```python
from build123d import *

# Parameters (mm, degrees)
BOSS_EXTRUDE1_DEPTH = 38.1
SKETCH2_W           = 19
SKETCH2_H           = 50
CUT_EXTRUDE1_DEPTH  = 2
CUT_EXTRUDE2_DEPTH  = 20


with BuildPart() as part:
    # Sketch1 → Boss-Extrude1 (new body)
    with BuildSketch(Plane(origin=(0, 0, 0), x_dir=(1, 0, 0), z_dir=(0, 1, 0))):
        Polygon((-138.61, 294.305), (350, -194.305), (350, -294.305), (-350, -294.305), (-350, 294.305), align=None)
    extrude(amount=BOSS_EXTRUDE1_DEPTH)

    # Sketch2 → Cut-Extrude1 (cut)
    with BuildSketch(Plane.XZ):
        with Locations((-340.5, -129.305)):
            Rectangle(SKETCH2_W, SKETCH2_H)
        with Locations((-340.5, 129.305)):
            Rectangle(SKETCH2_W, SKETCH2_H)
    extrude(amount=-CUT_EXTRUDE1_DEPTH, mode=Mode.SUBTRACT)

    # Sketch3 → Cut-Extrude2 (cut)
    with BuildSketch(Plane(origin=(0, 0, 0), x_dir=(1, 0, 0), z_dir=(0, 1, 0))):
        Polygon((-138.61, 294.305), (-181.946540118, 250.968459882), (-146.706941406, 216.891522613), (-104.668874503, 260.363874503), align=None)
    extrude(amount=CUT_EXTRUDE2_DEPTH, mode=Mode.SUBTRACT)


solid = part.part
```
CAD build for the part. Positions are in the model's coordinates, mm. A direction names the side the tool comes from. Round coordinates to 2 decimals unless told otherwise and drop trailing zeros. Write each loop counter-clockwise with the first axis right and the second up, starting at its lowest first coordinate (ties: lowest second). Pieces come first, ordered by that corner, then holes. Notation, with made-up numbers: (22.5, -18.5) -> (77.5, -18.5) arc R12 cw to (77.5, 2.5) -> close; hole circle Ø6 at (85, 81). An arc over 180 degrees is marked (long way). Answer in a Markdown table with one row per item. Add a question column.
Item 1: Drop flat-ended pins along their axis: pin 1 Ø10 at (y, z) = (19, -12.5) entering from +X (3 decimals); pin 2 Ø12 at (y, z) = (19, -177) entering from +X (3 decimals); pin 3 Ø1.6 at (y, z) = (1, 136.5) entering from -X. Give the stop position or say it passes through.
Item 2: Which spindle directions (+Z, -Z, +X, -X, +Y, -Y) get a long thin tool onto all of the face, cutting with end or side? Do faces 5 (the face through (-159.975, 9.86, -272.94)), 6 (the face through (-73, 0, 61)), 7 (the face through (-341, 2, 130)). Say none if no direction does.
Item 3: Mould opens along X. For faces 1 (the face through (102.275, 18.783, -53.42)), 2 (the face through (-164.573, 9.86, -234.169)), 3 (the face through (-350, 19, 4)), 4 (the face through (-246, 19, -294.305)) say: pulls with the +X half, pulls with the -X half, needs draft (parallel to the pull), parting line crosses it, or undercut.
Item 4: Saw through at D-D, the plane z = 0.5. Write the cut outline in (x, y) (3 decimals), then the cut area to 3 significant figures.
Item 5: Saw through at B-B, the plane z = -242. Write the cut outline in (x, y) (3 decimals), then the cut area to 3 significant figures.
Item 6: Drill centre lines: line 1 (Z direction, x = 198.5, y = 24) (3 decimals); line 2 (X direction, y = 17.5, z = 42.5) (3 decimals); line 3 (X direction, y = 30.5, z = 124) (3 decimals). Where is each one in solid material? Low to high. Write a range as from..to.
Item 7: Saw through at A-A, the plane y = 10.5. Write the cut outline in (x, z) (3 decimals), then the cut area to 3 significant figures.
Item 8: Saw through at C-C, the plane x = -96.5. Write the cut outline in (y, z) (3 decimals).
Findings below:
| question | item | result |
|---|---|---|
| 1 | pin 1 | stops at x = 148.195 |
| 1 | pin 2 | stops at x = -15.305 |
| 1 | pin 3 | stops at x = -331 |
| 2 | face 5 | -Y |
| 2 | face 6 | +Z, -Z, +X, -X, -Y |
| 2 | face 7 | -X, -Y |
| 3 | face 1 | pulls with the +X half |
| 3 | face 2 | undercut |
| 3 | face 3 | pulls with the -X half |
| 3 | face 4 | needs draft |
| 4 | outline | (-350, 0) -> (156.195, 0) -> (156.195, 38.1) -> (-350, 38.1) -> close |
| 4 | area | 19,300 mm^2 |
| 5 | outline | (-350, 0) -> (-172.672, 0) -> (-172.672, 20) -> (-122.427, 20) -> (-122.427, 0) -> (-86.305, 0) -> (-86.305, 38.1) -> (-350, 38.1) -> close |
| 5 | area | 9,040 mm^2 |
| 6 | line 1 | z = 42.805..294.305 |
| 6 | line 2 | x = -350..198.195 |
| 6 | line 3 | x = -350..279.695 |
| 7 | outline | (-350, -294.305) -> (-138.61, -294.305) -> (-181.947, -250.968) -> (-146.707, -216.892) -> (-104.669, -260.364) -> (350, 194.305) -> (350, 294.305) -> (-350, 294.305) -> close |
| 7 | area | 290,000 mm^2 |
| 8 | outline | (0, -252.195) -> (38.1, -252.195) -> (38.1, 294.305) -> (0, 294.305) -> close |
